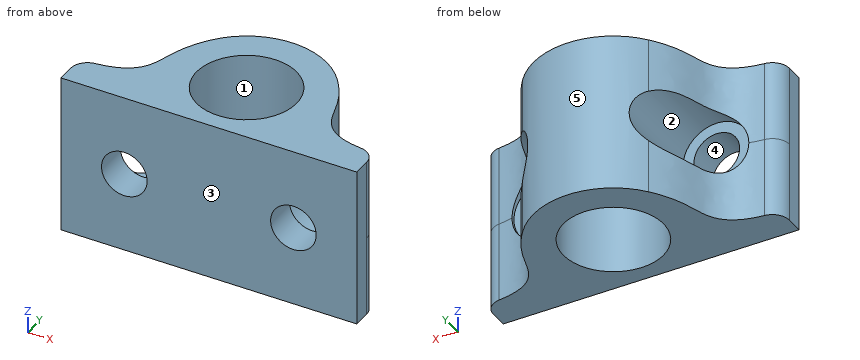
```python
from build123d import *

# Parameters (mm, degrees)
SKETCH1_R           = 7.5
BOSS_EXTRUDE1_DEPTH = 12
SKETCH3_R           = 3.425
CUT_EXTRUDE1_DEPTH  = 23.0000001
FILLET1_R           = 2.54
SKETCH4_R           = 5.08
CUT_EXTRUDE2_DEPTH  = 18.000000194


with BuildPart() as part:
    # Sketch1 → Boss-Extrude1 (new body, symmetric)
    with BuildSketch(Plane.XY):
        with BuildLine():
            Line((22.225, -10), (-22.225, -10))
            Line((-22.225, -10), (-22.225, -5))
            add(Edge.make_bspline(
                [(-22.225, -5), (-16.631079064, -4.98201906), (-12.322747723, -1.728386223), (-12.530535341, 3.440374129), (-9.467504716, 7.373354356)],
                knots=[0, 0, 0, 0, 0.501954987, 1, 1, 1, 1], degree=3))
            ThreePointArc((-9.467504716, 7.373354356), (0, 12), (9.467504716, 7.373354356))
            add(Edge.make_bspline(
                [(22.225, -5), (16.631079064, -4.98201906), (12.322747723, -1.728386223), (12.530535341, 3.440374129), (9.467504716, 7.373354356)],
                knots=[0, 0, 0, 0, 0.501954987, 1, 1, 1, 1], degree=3))
            Line((22.225, -5), (22.225, -10))
        make_face()
        Circle(SKETCH1_R, mode=Mode.SUBTRACT)
    extrude(amount=BOSS_EXTRUDE1_DEPTH, both=True)

    # Sketch3 → Cut-Extrude1 (cut, through all)
    with BuildSketch(Plane.XZ.offset(10)):
        with Locations((-12.7, 0)):
            Circle(SKETCH3_R)
        with Locations((12.7, 0)):
            Circle(SKETCH3_R)
    extrude(amount=-CUT_EXTRUDE1_DEPTH, mode=Mode.SUBTRACT)

    # Fillet1
    fillet1_edges = [part.edges().sort_by_distance(p)[0] for p in [
        (22.225, -5, -6),
        (-22.225, -5, 6),
    ]]
    fillet(fillet1_edges, radius=FILLET1_R)

    # Sketch4 → Cut-Extrude2 (cut, through all)
    with BuildSketch(Plane(origin=(0, -5.000000094, 0), x_dir=(-1, 0, 0), z_dir=(0, -1, 0))):
        with Locations((12.7, 0)):
            Circle(SKETCH4_R)
        with Locations((-12.7, 0)):
            Circle(SKETCH4_R)
    extrude(amount=-CUT_EXTRUDE2_DEPTH, mode=Mode.SUBTRACT)


solid = part.part
```
Geometry: final body of the model. Coordinates: model frame, mm. Face numbers are marked on the shaded views. A direction names the side the tool comes from. Coordinates: 2 decimals unless noted, no trailing zeros. Order: outer loops, then holes, each group sorted by start corner. A loop starts at its lowest first (then second) coordinate and runs counter-clockwise, first axis right, second up.
Item 1: Draft query along X for the marked faces 3, 4 and 5. Return one class per face: released by +X, released by -X, zero draft, split by the parting line, or undercut.
Answer:
face 3: zero draft
face 4: undercut
face 5: split by the parting line
Item 2: Access query for the marked faces 1 and 2. Directions: +Z, -Z, +X, -X, +Y, -Y. A direction counts if a zero-diameter tool reaches every point of the face in a straight line with its end or side. Return the directions, or none.
Answer:
face 1: +Z, -Z
face 2: +Y
Item 3: Contact query for flat-ended pins moving along their axis: P1, Ø6, axis at x = -12.7, z = 0, coming from the +Y side; P2, Ø1, axis at y = -6.5, z = -7.5, coming from the -X side; P3, Ø10, axis at x = 5.5, z = 6, coming from the +Y side; P4, Ø2, axis at y = -0.5, z = 6.5, coming from the +X side. Output: stop coordinate, or through.
Answer:
P1: passes through
P2: stops at x = -22.19
P3: stops at y = 11.99
P4: stops at x = 13.58
Item 4: Section query A-A (x = 0). Output: boundary loops of the cut face in (y, z).
Answer:
outline: (-10, -12) - (-7.5, -12) - (-7.5, 12) - (-10, 12) - close; (7.5, -12) - (12, -12) - (12, 12) - (7.5, 12) - close
Item 5: Material intervals for line 1 along Z through (x, y) = (-12.7, -6.1) (3 decimals); line 2 along Y through (x, z) = (-5.5, 0); line 3 along Z through (x, y) = (-14, -6.25), sorted ascending.
Answer:
line 1: z = -12 to -3.425, 3.425 to 12
line 2: y = -10 to -5.1, 5.1 to 10.67
line 3: z = -12 to -3.17, 3.17 to 12
Item 6: Section query B-B (z = -1.5). State how many separate pieces and enclosed holes the cut face has, then the cut area to 3 significant figures.
Answer:
separate pieces: 3
enclosed holes: 1
area: 236 mm2
